The listing builds one solid part. Answer for the finished solid, in the listing's coordinates (mm). A direction names the side the tool comes from. Give positions to 0.01 mm unless a question says otherwise; leave off trailing zeros. Order: outer loops, then holes, each group sorted by start corner. A loop starts at its lowest first (then second) coordinate and runs counter-clockwise, first axis right, second up.
```python
from build123d import *

# Parameters (mm, degrees)
BOSS_EXTRUDE4_DEPTH = 16.5
CUT_EXTRUDE2_DEPTH  = 1.5
CUT_EXTRUDE4_DEPTH  = 17.5
SKETCH6_W           = 12
SKETCH6_H           = 2
CUT_EXTRUDE5_DEPTH  = 17.5
BOSS_EXTRUDE5_DEPTH = 2
SKETCH10_R          = 2.38125
CUT_EXTRUDE6_DEPTH  = 13.606601718
CUT_EXTRUDE7_DEPTH  = 17.5
SKETCH12_R          = 2.38125
CUT_EXTRUDE8_DEPTH  = 6.35
SKETCH13_W          = 6.5
SKETCH13_H          = 9
CUT_EXTRUDE11_DEPTH = 2
SKETCH15_W          = 16.5
SKETCH15_H          = 2
CUT_EXTRUDE13_DEPTH = 18
SKETCH16_W          = 2
SKETCH16_H          = 35.1
BOSS_EXTRUDE6_DEPTH = 5


with BuildPart() as part:
    # Sketch1 → Boss-Extrude4 (new body)
    with BuildSketch(Plane(origin=(0, 0, 0), x_dir=(0, 0, -1), z_dir=(1, 0, 0))):
        Polygon((0, 0), (0, 37.1), (-10.606601718, 47.706601718), (12, 47.706601718), (12, 0), align=None)
    extrude(amount=BOSS_EXTRUDE4_DEPTH)

    # Sketch4 → Cut-Extrude2 (cut)
    with BuildSketch(Plane.ZY):
        Polygon((0, 37.1), (0, 47.706601718), (10.606601718, 47.706601718), align=None)
    extrude(amount=-CUT_EXTRUDE2_DEPTH, mode=Mode.SUBTRACT)

    # Sketch5 → Cut-Extrude4 (cut, through all)
    with BuildSketch(Plane(origin=(16.5, 0, 0), x_dir=(0, 0, -1), z_dir=(1, 0, 0))):
        Polygon((-3.566952421, 40.666952421), (-2.859845639, 39.959845639), (-1.799185468, 41.020505811), (0, 39.221320344), (0, 42.756854249), (-2.683068944, 45.439923194), (-4.450835897, 43.672156241), (-3.036622335, 42.257942678), (-4.097282506, 41.197282506), align=None)
    extrude(amount=-CUT_EXTRUDE4_DEPTH, mode=Mode.SUBTRACT)

    # Sketch6 → Cut-Extrude5 (cut, through all)
    with BuildSketch(Plane(origin=(16.5, 0, 0), x_dir=(0, 0, -1), z_dir=(1, 0, 0))):
        with Locations((6, 1)):
            Rectangle(SKETCH6_W, SKETCH6_H)
    extrude(amount=-CUT_EXTRUDE5_DEPTH, mode=Mode.SUBTRACT)

    # Sketch9 → Boss-Extrude5 (add)
    with BuildSketch(Plane.XY):
        with BuildLine():
            Line((16.5, 29), (16.5, 25))
            Line((16.5, 25), (20.518219338, 25))
            ThreePointArc((20.518219338, 25), (24.518219338, 29), (20.518219338, 33))
            Line((20.518219338, 33), (16.5, 33))
            Line((16.5, 33), (16.5, 29))
        make_face()
    extrude(amount=-BOSS_EXTRUDE5_DEPTH)

    # Sketch10 → Cut-Extrude6 (cut, through all)
    with BuildSketch(Plane(origin=(0, 0, -2), x_dir=(-1, 0, 0), z_dir=(0, 0, -1))):
        with Locations((-20.518219338, 29)):
            Circle(SKETCH10_R)
    extrude(amount=-CUT_EXTRUDE6_DEPTH, mode=Mode.SUBTRACT)

    # Sketch11 → Cut-Extrude7 (cut, through all)
    with BuildSketch(Plane(origin=(16.5, 0, 0), x_dir=(0, 0, -1), z_dir=(1, 0, 0))):
        Polygon((0, 37.1), (-10.606601718, 47.706601718), (12, 47.706601718), (12, 37.1), align=None)
    extrude(amount=-CUT_EXTRUDE7_DEPTH, mode=Mode.SUBTRACT)

    # Sketch12 → Cut-Extrude8 (cut)
    with BuildSketch(Plane.XZ.offset(-2)):
        with Locations((8.25, -6)):
            Circle(SKETCH12_R)
    extrude(amount=-CUT_EXTRUDE8_DEPTH, mode=Mode.SUBTRACT)

    # Sketch13 → Cut-Extrude11 (cut)
    with BuildSketch(Plane.XY):
        with Locations((6.25, 25.5)):
            Rectangle(SKETCH13_W, SKETCH13_H)
    extrude(amount=-CUT_EXTRUDE11_DEPTH, mode=Mode.SUBTRACT)

    # Sketch15 → Cut-Extrude13 (cut)
    with BuildSketch(Plane(origin=(0, 37.1, 0), x_dir=(1, 0, 0), z_dir=(0, 1, 0))):
        with Locations((8.25, 3)):
            Rectangle(SKETCH15_W, SKETCH15_H)
    extrude(amount=-CUT_EXTRUDE13_DEPTH, mode=Mode.SUBTRACT)

    # Sketch16 → Boss-Extrude6 (add)
    with BuildSketch(Plane.ZY):
        with Locations((-1, 19.55)):
            Rectangle(SKETCH16_W, SKETCH16_H)
    extrude(amount=BOSS_EXTRUDE6_DEPTH)


solid = part.part
```
1) Find section B-B (x = 8.25). Write down the section's boundary in (y, z).
Geometry says:
outline: (2, -12) - (37.1, -12) - (37.1, -4) - (19.1, -4) - (19.1, -2) - (21, -2) - (21, 0) - (2, 0) - (2, -3.62) - (8.35, -3.62) - (8.35, -8.38) - (2, -8.38) - close; (30, -2) - (37.1, -2) - (37.1, 0) - (30, 0) - close
2) Find section D-D (y = 6). Write down the section's boundary in (x, z), then the cut area to 3 significant figures.
Geometry says:
outline: (-5, -2) - (0, -2) - (0, -12) - (16.5, -12) - (16.5, 0) - (-5, 0) - close; hole circle Ø4.76 at (8.25, -6)
area: 190 mm2
3) For a pull along Z with two mould halves and no side action, classify faces 6 (the flat face through (19, 33, -1)), 7 (the flat face through (8, 20, -12)), 8 (the flat face through (8, 28, -4)) as +Z half, -Z half, draft (parallel to the pull), parting line (faces both ways), or undercut.
Geometry says:
face 6: draft
face 7: -Z half
face 8: undercut
4) Given P1, Ø1.5, axis at y = 32.5, z = -6, coming from the -X side; P2, Ø1, axis at y = 35.5, z = -0.5, coming from the +X side; P3, Ø1, axis at x = 19.5, z = -1.5, coming from the +Y side, each flat-ended and moving along its own axis, determine where each tip first touches the part or whether it passes through.
Geometry says:
P1: stops at x = 0
P2: stops at x = 16.5
P3: stops at y = 33
5) Straight lines are drawn through the part: probe 1 along Z at (x, y) = (5, 33.5); probe 2 along Z at (x, y) = (8.25, 5.5); probe 3 along Y at (x, z) = (7, -4.75). For each, find the intervals that lie inside material, in ascending order.
Geometry says:
probe 1: z = -12 to -4, -2 to 0
probe 2: z = -12 to -8.38, -3.62 to 0
probe 3: y = 8.35 to 37.1
6) Find section A-A (y = 29). Write down the section's boundary in (x, z).
Geometry says:
outline: (-5, -2) - (3, -2) - (3, 0) - (-5, 0) - close; (0, -12) - (16.5, -12) - (16.5, -4) - (0, -4) - close; (9.5, -2) - (18.14, -2) - (18.14, 0) - (9.5, 0) - close; (22.9, -2) - (24.52, -2) - (24.52, 0) - (22.9, 0) - close
7) Find section C-C (z = -1). Write down the section's boundary in (x, y).
Geometry says:
outline: (-5, 2) - (16.5, 2) - (16.5, 25) - (20.52, 25) arc R4 ccw to (20.52, 33) - (16.5, 33) - (16.5, 37.1) - (-5, 37.1) - close; hole (3, 21) - (9.5, 21) - (9.5, 30) - (3, 30) - close; hole circle Ø4.76 at (20.52, 29)
8) A tool of negligible diameter and unlimited length cuts with its end or side. For faces 1 (the cylindrical face through (5.87, 5.13, -5.9)), 2 (the flat face through (8, 19.1, -3)), 3 (the flat face through (18, 25, -1)), 4 (the flat face through (16.5, 35, -1)), 5 (the flat face through (9.5, 25, -1)), from which of +Z, -Z, +X, -X, +Y, -Y can it reach the whole face along a straight path? Write none if from no direction.
Geometry says:
face 1: -Y
face 2: +X, -X, +Y
face 3: +Z, -Z, +X, -Y
face 4: +Z, -Z, +X, +Y
face 5: +Z
